Build history of the part. All positions in model axes, mm. Give positions to 0.01 mm unless a question says otherwise; leave off trailing zeros. Loops run counter-clockwise (first coordinate to the right, second up) from the corner with the lowest first, then second, coordinate; pieces in that order, holes last. Notation, with made-up numbers: M 34,-15.5 L 43,-15.5 A27 cw 43,21.5 Z; hole C 26.5,-0.5 d10. An arc over 180 degrees is marked long. Answer in a Markdown table with one row per item. Add a question column.
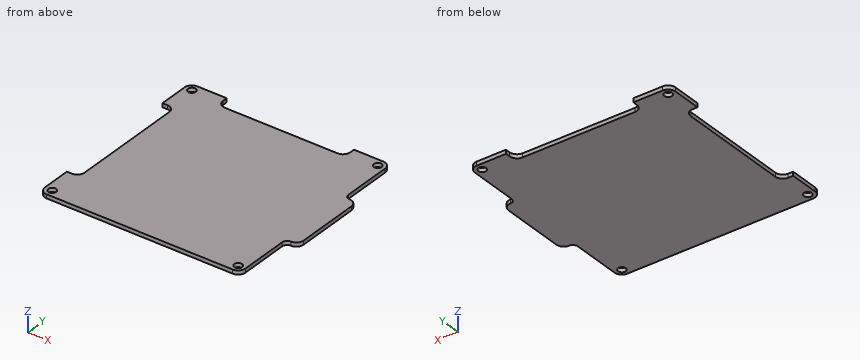
```python
from build123d import *

# Parameters (mm, degrees)
BOSS_EXTRUDE1_DEPTH        = 1.6
F_3_2_3_2_DIAMETER_HOLE1_D = 3.2
FILLET1_R                  = 3
FILLET3_R                  = 2


with BuildPart() as part:
    # Sketch1 → Boss-Extrude1 (new body)
    with BuildSketch(Plane.XY):
        Polygon((-15.5, 86.75), (-15.5, 81.75), (-67.5, 81.75), (-67.5, 86.75), (-82.5, 86.75), (-82.5, 71.75), (-77.5, 71.75), (-77.5, 19.75), (-82.5, 19.75), (-82.5, 4.75), (-0.5, 4.75), (-0.5, 29.75), (4.5, 29.75), (4.5, 61.75), (-0.5, 61.75), (-0.5, 86.75), align=None)
    extrude(amount=-BOSS_EXTRUDE1_DEPTH)

    # Ø3.2 (3.2) Diameter Hole1 (through all)
    with Locations(Plane(origin=(0, 0, -1.6), x_dir=(-1, 0, 0), z_dir=(0, 0, -1))):
        with Locations((3.5, 83.75), (3.5, 7.75), (79.5, 7.75), (79.5, 83.75)):
            Hole(F_3_2_3_2_DIAMETER_HOLE1_D / 2)

    # Fillet1
    fillet1_edges = [part.edges().sort_by_distance(p)[0] for p in [
        (4.5, 61.75, -0.8),
        (4.5, 29.75, -0.8),
        (-0.5, 4.75, -0.8),
        (-82.5, 4.75, -0.8),
        (-77.5, 19.75, -0.8),
        (-77.5, 71.75, -0.8),
        (-82.5, 86.75, -0.8),
        (-67.5, 81.75, -0.8),
        (-15.5, 81.75, -0.8),
        (-0.5, 86.75, -0.8),
    ]]
    fillet(fillet1_edges, radius=FILLET1_R)

    # Fillet3
    fillet3_edges = [part.edges().sort_by_distance(p)[0] for p in [
        (-0.5, 29.75, -0.8),
        (-0.5, 61.75, -0.8),
    ]]
    fillet(fillet3_edges, radius=FILLET3_R - 0.0001)  # a hair under: the kernel refuses the full size


solid = part.part
```
(1) Slice it at A-A, the plane z = -0.5. State how many separate pieces and enclosed holes the cut face has, then the cut area to 3 significant figures.
(2) Pin check, flat tips, straight feed: pin 1 (0.8 mm diameter, centred on x = -81.5, z = -0.5, fed in from +Y); pin 2 (3 mm diameter, centred on x = -79.5, y = 7.75, fed in from -Z); pin 3 (0.8 mm diameter, centred on y = 85.5, z = -1, fed in from -X); pin 4 (0.5 mm diameter, centred on y = 86, z = -1, fed in from +X). Stop position of each tip, or through.
(3) Slice it at B-B, the plane y = 42. Give the cut face in (x, z), then the cut area to 3 significant figures.
(4) Slice it at C-C, the plane x = -30.5. Give the cut face in (y, z).
(5) Wall check: line 1 (X direction, y = 83, z = -0.55); line 2 (X direction, y = 83.75, z = -1.05); line 3 (Y direction, x = -19.5, z = -0.5). Give the ranges that are in metal, low to high.
Solution:
| question | item | result |
|---|---|---|
| 1 | separate pieces | 1 |
| 1 | enclosed holes | 4 |
| 1 | area | 6,330 mm^2 |
| 2 | pin 1 | y = 86.29 |
| 2 | pin 2 | through |
| 2 | pin 3 | x = -82.18 |
| 2 | pin 4 | x = -1.26 |
| 3 | outline | M -77.5,-1.6 L 4.5,-1.6 L 4.5,0 L -77.5,0 Z |
| 3 | area | 131 mm^2 |
| 4 | outline | M 4.75,-1.6 L 81.75,-1.6 L 81.75,0 L 4.75,0 Z |
| 5 | line 1 | -82.5 to -80.91, -78.09 to -66.94, -16.06 to -4.91, -2.09 to -0.5 |
| 5 | line 2 | -82.5 to -81.1, -77.9 to -67.33, -15.67 to -5.1, -1.9 to -0.5 |
| 5 | line 3 | 4.75 to 81.75 |
